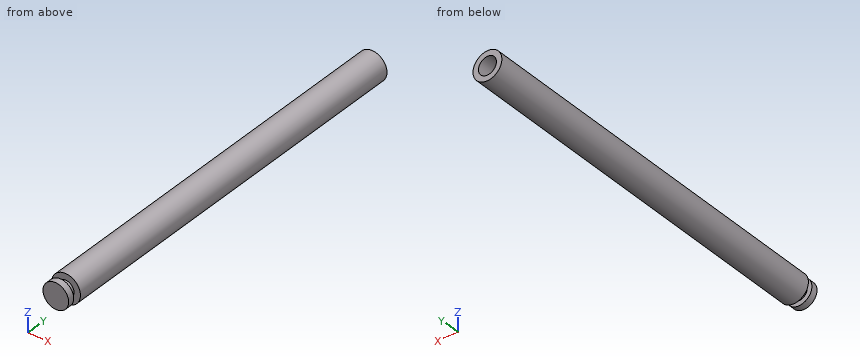
```python
from build123d import *

# Parameters (mm, degrees)
SKETCH1_R           = 2.25
BOSS_EXTRUDE1_DEPTH = 60
SKETCH1_3_R         = 1.375
BOSS_EXTRUDE2_DEPTH = 1
SKETCH5_R           = 1.25
BOSS_EXTRUDE3_DEPTH = 1
SKETCH6_R           = 2
BOSS_EXTRUDE4_DEPTH = 1
SKETCH12_R          = 1.4
CUT_EXTRUDE1_DEPTH  = 15


with BuildPart() as part:
    # Sketch1 → Boss-Extrude1 (new body)
    with BuildSketch(Plane(origin=(0, 0, 0), x_dir=(1, 0, 0), z_dir=(0, 1, 0))):
        with Locations((-0.522013312, 0.511138034)):
            Circle(SKETCH1_R)
    extrude(amount=BOSS_EXTRUDE1_DEPTH)

    # Sketch1<3> → Boss-Extrude2 (add)
    with BuildSketch(Plane(origin=(0, 0, 0), x_dir=(1, 0, 0), z_dir=(0, 1, 0))):
        with Locations((-0.522013312, 0.511138034)):
            Circle(SKETCH1_3_R)
    extrude(amount=BOSS_EXTRUDE2_DEPTH)

    # Sketch5 → Boss-Extrude3 (add)
    with BuildSketch(Plane.XZ):
        with Locations((-0.522013312, -0.511138034)):
            Circle(SKETCH5_R)
    extrude(amount=BOSS_EXTRUDE3_DEPTH)

    # Sketch6 → Boss-Extrude4 (add)
    with BuildSketch(Plane.XZ.offset(1)):
        with Locations((-0.522013312, -0.511138034)):
            Circle(SKETCH6_R)
    extrude(amount=BOSS_EXTRUDE4_DEPTH)

    # Sketch12 → Cut-Extrude1 (cut)
    with BuildSketch(Plane(origin=(0, 60, 0), x_dir=(1, 0, 0), z_dir=(0, 1, 0))):
        with Locations((-0.522013312, 0.511138034)):
            Circle(SKETCH12_R)
    extrude(amount=-CUT_EXTRUDE1_DEPTH, mode=Mode.SUBTRACT)


solid = part.part
```
Design review of the part built by this model. Coordinates are the model's own, in mm. Coordinates: 2 decimals unless noted, no trailing zeros. Write each loop counter-clockwise with the first axis right and the second up, starting at its lowest first coordinate (ties: lowest second). Pieces come first, ordered by that corner, then holes.
1) Add section D-D (y = 48). Write out the cut boundary in (x, z), plus the area to 3 significant figures.
2) Add section A-A (x = -0.55). Write out the cut boundary in (y, z).
3) Add section B-B (z = 0.1). Write out the cut boundary in (x, y), plus the area to 3 significant figures.
4) Insertion check: pin 1 (1.4 mm diameter, centred on x = -1, z = -0.5, fed in from +Y); pin 2 (1 mm diameter, centred on x = -2.5, y = 19.5, fed in from +Z). Each pin has a flat end and moves straight along its axis. Give the tip position at first contact, or say it passes through.
5) To check wall thickness, follow L1, parallel to Y at x = -1.5, z = -2.2; L2, parallel to Y at x = -1.3, z = -1.55; L3, parallel to Z at x = -0.55, y = 54. State the ranges of each line that lie inside material, in increasing order.
6) Add section C-C (y = 7.5). Write out the cut boundary in (x, z).
Check result:
1. outline: circle Ø4.5 at (-0.52, -0.51); hole circle Ø2.8 at (-0.52, -0.51)
1. area: 9.75 mm2
2. outline: (-2, -2.51) - (-1, -2.51) - (-1, -1.76) - (0, -1.76) - (0, -2.76) - (60, -2.76) - (60, -1.91) - (45, -1.91) - (45, 0.89) - (60, 0.89) - (60, 1.74) - (0, 1.74) - (0, 0.74) - (-1, 0.74) - (-1, 1.49) - (-2, 1.49) - close
3. outline: (-2.69, 0) - (-1.61, 0) - (-1.61, -1) - (-2.43, -1) - (-2.43, -2) - (1.38, -2) - (1.38, -1) - (0.57, -1) - (0.57, 0) - (1.64, 0) - (1.64, 60) - (0.74, 60) - (0.74, 45) - (-1.78, 45) - (-1.78, 60) - (-2.69, 60) - close
3. area: 228 mm2
4. pin 1: stops at y = 45
4. pin 2: stops at z = 1.19
5. L1: y = -2 to -1, 0 to 60
5. L2: y = -2 to -1, 0 to 45
5. L3: z = -2.76 to -1.91, 0.89 to 1.74
6. outline: circle Ø4.5 at (-0.52, -0.51)
